```python
from build123d import *

# Parameters (mm, degrees)
ESBO_O1_W                   = 140
ESBO_O1_H                   = 95
RESSALTO_EXTRUS_O1_DEPTH    = 1.5
ESBO_O2_R                   = 1.5
ESBO_O2_W                   = 40
ESBO_O2_H                   = 3
CORTE_EXTRUS_O1_DEPTH       = 85.647799735
ESBO_O3_W                   = 3
ESBO_O3_H                   = 31
ESBO_O3_W_2                 = 30
ESBO_O3_H_2                 = 3
RESSALTO_EXTRUS_O2_DEPTH    = 3
CORTE_EXTRUS_O11_DEPTH      = 89.815820663
CORTE_EXTRUS_O11_DEPTH_BACK = 89.815820663
ESBO_O30_R                  = 4
CORTE_EXTRUS_O12_DEPTH      = 89.815820663
CORTE_EXTRUS_O12_DEPTH_BACK = 89.815820663
ESBO_O31_R                  = 1.5
CORTE_EXTRUS_O2_DEPTH       = 89.815820663
CUT_EXTRUDE2_DEPTH          = 89.777812543
CUT_EXTRUDE2_DEPTH_BACK     = 89.777812543
CUT_EXTRUDE6_DEPTH          = 89.815820663
CUT_EXTRUDE6_DEPTH_BACK     = 89.815820663
CUT_EXTRUDE8_DEPTH          = 89.777812543
CUT_EXTRUDE8_DEPTH_BACK     = 89.777812543
CUT_EXTRUDE9_DEPTH          = 89.815820663
CUT_EXTRUDE12_DEPTH         = 89.777812543
CUT_EXTRUDE12_DEPTH_BACK    = 89.777812543
SKETCH16_R                  = 1.5
FILLET1_R                   = 5


with BuildPart() as part:
    # Esboço1 → Ressalto-extrusão1 (new, symmetric)
    with BuildSketch(Plane.XY):
        Rectangle(ESBO_O1_W, ESBO_O1_H)
    extrude(amount=RESSALTO_EXTRUS_O1_DEPTH, both=True)

    # Esboço2 → Corte-extrusão1 (cut, through all)
    with BuildSketch(Plane.XY.offset(1.5)):
        with Locations((-31.5, -1)):
            Circle(ESBO_O2_R)
        with Locations(Location((31.5, -1, 0), (0, 0, 180))):
            Circle(ESBO_O2_R)
        with Locations((0, -46)):
            Rectangle(ESBO_O2_W, ESBO_O2_H)
        with Locations((0, -1)):
            Rectangle(ESBO_O2_W, ESBO_O2_H)
    extrude(amount=-CORTE_EXTRUS_O1_DEPTH, mode=Mode.SUBTRACT)

    # Esboço3 → Ressalto-extrusão2 (add, through all)
    with BuildSketch(Plane.XY.offset(1.5)):
        with Locations((71.5, 0)):
            Rectangle(ESBO_O3_W, ESBO_O3_H)
        with Locations((-71.5, 0)):
            Rectangle(ESBO_O3_W, ESBO_O3_H)
        with Locations((-35, 49)):
            Rectangle(ESBO_O3_W_2, ESBO_O3_H_2)
        with Locations((35, 49)):
            Rectangle(ESBO_O3_W_2, ESBO_O3_H_2)
    extrude(amount=-RESSALTO_EXTRUS_O2_DEPTH)

    # Esboço30 → Corte-extrusão11 (cut, two sides: drawn at the far end of the back side and taken through both)
    with BuildSketch(Plane(origin=(0, 0, -1.5), x_dir=(-1, 0, 0), z_dir=(0, 0, -1)).offset(-CORTE_EXTRUS_O11_DEPTH_BACK)):
        with Locations((55, -28.5)):
            Circle(ESBO_O30_R)
    extrude(amount=CORTE_EXTRUS_O11_DEPTH + CORTE_EXTRUS_O11_DEPTH_BACK, mode=Mode.SUBTRACT)

    # Esboço31 → Corte-extrusão12 (cut, two sides: drawn at the far end of the back side and taken through both)
    with BuildSketch(Plane(origin=(0, 0, -1.5), x_dir=(-1, 0, 0), z_dir=(0, 0, -1)).offset(-CORTE_EXTRUS_O12_DEPTH_BACK)):
        with Locations((64, -19.5)):
            Circle(ESBO_O31_R)
        with Locations((64, -37.5)):
            Circle(ESBO_O31_R)
        with Locations((31, -19.5)):
            Circle(ESBO_O31_R)
        with Locations((31, -37.5)):
            Circle(ESBO_O31_R)
    extrude(amount=CORTE_EXTRUS_O12_DEPTH + CORTE_EXTRUS_O12_DEPTH_BACK, mode=Mode.SUBTRACT)

    # Esboço4 → Corte-extrusão2 (cut, through all)
    with BuildSketch(Plane.XY.offset(1.5)):
        with BuildLine():
            Line((40, -26.5), (46, -26.5))
            ThreePointArc((46, -26.5), (48, -28.5), (46, -30.5))
            Line((46, -30.5), (40, -30.5))
            ThreePointArc((40, -30.5), (38, -28.5), (40, -26.5))
        make_face()
    extrude(amount=-CORTE_EXTRUS_O2_DEPTH, mode=Mode.SUBTRACT)

    # Sketch5 → Cut-Extrude2 (cut, two sides: drawn at the far end of the back side and taken through both)
    with BuildSketch(Plane.XY.offset(-CUT_EXTRUDE2_DEPTH_BACK)):
        with BuildLine():
            Line((-1.5, -44.5), (1.5, -44.5))
            Line((1.5, -44.5), (1.5, -40.5))
            Line((1.5, -40.5), (2.85, -40.5))
            Line((2.85, -40.5), (2.85, -38.23))
            Line((2.85, -38.23), (1.5, -38.23))
            Line((1.5, -38.23), (1.5, -33.5))
            ThreePointArc((1.5, -33.5), (1.207106781, -32.792893219), (0.5, -32.5))
            Line((0.5, -32.5), (-0.5, -32.5))
            ThreePointArc((-0.5, -32.5), (-1.207106781, -32.792893219), (-1.5, -33.5))
            Line((-1.5, -33.5), (-1.5, -38.23))
            Line((-1.5, -38.23), (-2.85, -38.23))
            Line((-2.85, -38.23), (-2.85, -40.5))
            Line((-2.85, -40.5), (-1.5, -40.5))
            Line((-1.5, -40.5), (-1.5, -44.5))
        make_face()
    extrude(amount=CUT_EXTRUDE2_DEPTH + CUT_EXTRUDE2_DEPTH_BACK, mode=Mode.SUBTRACT)

    # Sketch8 → Cut-Extrude6 (cut, two sides: drawn at the far end of the back side and taken through both)
    with BuildSketch(Plane.XY.offset(1.5).offset(-CUT_EXTRUDE6_DEPTH_BACK)):
        with BuildLine():
            Line((-56, 39.75), (-56, 26.75))
            ThreePointArc((-56, 26.75), (-56.439339828, 25.689339828), (-57.5, 25.25))
            Line((-57.5, 25.25), (-60.5, 25.25))
            ThreePointArc((-60.5, 25.25), (-61.560660172, 24.810660172), (-62, 23.75))
            Line((-62, 23.75), (-62, 23.5))
            ThreePointArc((-62, 23.5), (-63.5, 22), (-65, 23.5))
            Line((-65, 23.5), (-65, 23.75))
            ThreePointArc((-65, 23.75), (-65.24500996, 24.571583836), (-65.9, 25.124772708))
            ThreePointArc((-65.9, 25.124772708), (-66.336660027, 25.49356529), (-66.5, 26.041287847))
            Line((-66.5, 26.041287847), (-66.5, 40.458712153))
            ThreePointArc((-66.5, 40.458712153), (-66.336660027, 41.00643471), (-65.9, 41.375227292))
            ThreePointArc((-65.9, 41.375227292), (-65.24500996, 41.928416164), (-65, 42.75))
            Line((-65, 42.75), (-65, 43))
            ThreePointArc((-65, 43), (-63.5, 44.5), (-62, 43))
            Line((-62, 43), (-62, 42.75))
            ThreePointArc((-62, 42.75), (-61.560660172, 41.689339828), (-60.5, 41.25))
            Line((-60.5, 41.25), (-57.5, 41.25))
            ThreePointArc((-57.5, 41.25), (-56.439339828, 40.810660172), (-56, 39.75))
        make_face()
        with BuildLine():
            Line((56, 39.75), (56, 26.75))
            ThreePointArc((56, 26.75), (56.439339828, 25.689339828), (57.5, 25.25))
            Line((57.5, 25.25), (60.5, 25.25))
            ThreePointArc((60.5, 25.25), (61.560660172, 24.810660172), (62, 23.75))
            Line((62, 23.75), (62, 23.5))
            ThreePointArc((62, 23.5), (63.5, 22), (65, 23.5))
            Line((65, 23.5), (65, 23.75))
            ThreePointArc((65, 23.75), (65.24500996, 24.571583836), (65.9, 25.124772708))
            ThreePointArc((65.9, 25.124772708), (66.336660027, 25.49356529), (66.5, 26.041287847))
            Line((66.5, 26.041287847), (66.5, 40.458712153))
            ThreePointArc((66.5, 40.458712153), (66.336660027, 41.00643471), (65.9, 41.375227292))
            ThreePointArc((65.9, 41.375227292), (65.24500996, 41.928416164), (65, 42.75))
            Line((65, 42.75), (65, 43))
            ThreePointArc((65, 43), (63.5, 44.5), (62, 43))
            Line((62, 43), (62, 42.75))
            ThreePointArc((62, 42.75), (61.560660172, 41.689339828), (60.5, 41.25))
            Line((60.5, 41.25), (57.5, 41.25))
            ThreePointArc((57.5, 41.25), (56.439339828, 40.810660172), (56, 39.75))
        make_face()
    extrude(amount=CUT_EXTRUDE6_DEPTH + CUT_EXTRUDE6_DEPTH_BACK, mode=Mode.SUBTRACT)

    # Sketch11 → Cut-Extrude8 (cut, two sides: drawn at the far end of the back side and taken through both)
    with BuildSketch(Plane.XY.offset(-CUT_EXTRUDE8_DEPTH_BACK)):
        with BuildLine():
            Line((-36.5, 50.5), (-33.5, 50.5))
            Line((-33.5, 50.5), (-33.5, 46.5))
            Line((-33.5, 46.5), (-32.15, 46.5))
            Line((-32.15, 46.5), (-32.15, 44.23))
            Line((-32.15, 44.23), (-33.5, 44.23))
            Line((-33.5, 44.23), (-33.5, 39.5))
            ThreePointArc((-33.5, 39.5), (-33.792893219, 38.792893219), (-34.5, 38.5))
            Line((-34.5, 38.5), (-35.5, 38.5))
            ThreePointArc((-35.5, 38.5), (-36.207106781, 38.792893219), (-36.5, 39.5))
            Line((-36.5, 39.5), (-36.5, 44.23))
            Line((-36.5, 44.23), (-37.85, 44.23))
            Line((-37.85, 44.23), (-37.85, 46.5))
            Line((-37.85, 46.5), (-36.5, 46.5))
            Line((-36.5, 46.5), (-36.5, 50.5))
        make_face()
    extrude(amount=CUT_EXTRUDE8_DEPTH + CUT_EXTRUDE8_DEPTH_BACK, mode=Mode.SUBTRACT)

    # Sketch12 → Cut-Extrude9 (cut, through all)
    with BuildSketch(Plane.XY.offset(1.5)):
        with BuildLine():
            Line((-1.5, 20), (-1.5, 35))
            ThreePointArc((-1.5, 35), (0, 36.5), (1.5, 35))
            Line((1.5, 35), (1.5, 20))
            ThreePointArc((1.5, 20), (0, 18.5), (-1.5, 20))
        make_face()
    extrude(amount=-CUT_EXTRUDE9_DEPTH, mode=Mode.SUBTRACT)

    # Sketch16 → Cut-Extrude12 (cut, two sides: drawn at the far end of the back side and taken through both)
    with BuildSketch(Plane.XY.offset(-CUT_EXTRUDE12_DEPTH_BACK)):
        with Locations((-12.5, 15.35)):
            Circle(SKETCH16_R)
        with Locations((12.5, 15.35)):
            Circle(SKETCH16_R)
        with Locations((-12.5, -8.95)):
            Circle(SKETCH16_R)
        with Locations((12.5, -8.95)):
            Circle(SKETCH16_R)
        with BuildLine():
            Line((10.5, 13.35), (14.5, 13.35))
            ThreePointArc((14.5, 13.35), (15.207106781, 13.057106781), (15.5, 12.35))
            Line((15.5, 12.35), (15.5, 4.15))
            ThreePointArc((15.5, 4.15), (15.207106781, 3.442893219), (14.5, 3.15))
            Line((14.5, 3.15), (10.5, 3.15))
            ThreePointArc((10.5, 3.15), (9.792893219, 3.442893219), (9.5, 4.15))
            Line((9.5, 4.15), (9.5, 12.35))
            ThreePointArc((9.5, 12.35), (9.792893219, 13.057106781), (10.5, 13.35))
        make_face()
    extrude(amount=CUT_EXTRUDE12_DEPTH + CUT_EXTRUDE12_DEPTH_BACK, mode=Mode.SUBTRACT)

    # Fillet1
    fillet1_edges = [part.edges().sort_by_distance(p)[0] for p in [
        (-70, 47.5, 0),
        (70, 47.5, 0),
    ]]
    fillet(fillet1_edges, radius=FILLET1_R)


solid = part.part
```
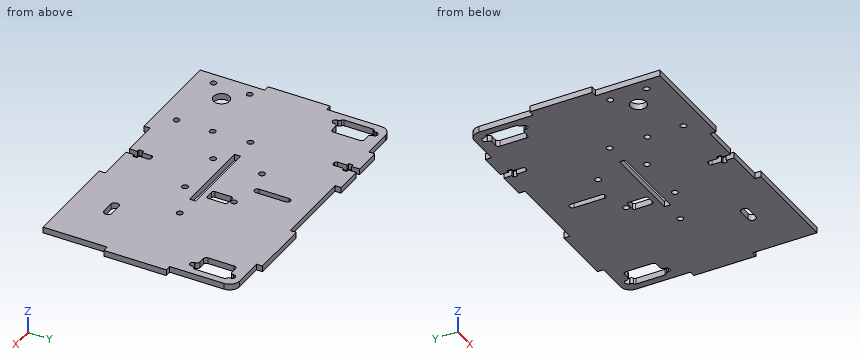
Geometry: final body of the model. Coordinates: model frame, mm. Round coordinates to 2 decimals unless told otherwise and drop trailing zeros. Order: outer loops, then holes, each group sorted by start corner. A loop starts at its lowest first (then second) coordinate and runs counter-clockwise, first axis right, second up. Notation, with made-up numbers: M -25,40.5 L -18,40.5 A32 ccw -18,71.5 Z; hole C 71,64.25 d11. An arc over 180 degrees is marked long. Use one line per item in the form item = value. Start each with the question number.
Q1. Cut plane D-D (z = -0.7). Count the separate pieces of the cut face and the enclosed holes in it, and give its area (3 significant figures).
Q2. Pin query (flat end, axial travel): pin 1 Ø0.9 at (y, z) = (42.5, 0) entering from +X; pin 2 Ø1.1 at (x, z) = (0, 0) entering from -Y; pin 3 Ø1.5 at (y, z) = (49, 0) entering from -X. Return the tip coordinate at first contact, or that it passes through.
Q3. Cut plane A-A (y = -28.5). Return loops of the section in (x, z), and give its area (3 significant figures).
Q4. Cut plane C-C (x = -12.5). Return loops of the section in (y, z).
Q5. Cut plane B-B (x = 42). Return loops of the section in (y, z).
Q6. Material intervals for line 1 (X direction, y = -8.95, z = 0.25); line 2 (X direction, y = 34, z = -1.1); line 3 (Y direction, x = -6.5, z = 0.3), sorted ascending. Write a range as [from, to].
Geometry results:
q1.separate_pieces = 1
q1.enclosed_holes = 17
q1.area = 12,700 mm^2
q2.pin_1 = 70
q2.pin_2 = -32.5
q2.pin_3 = -50
q3.outline = M -70,-1.5 L -59,-1.5 L -59,1.5 L -70,1.5 Z; M -51,-1.5 L 38,-1.5 L 38,1.5 L -51,1.5 Z; M 48,-1.5 L 70,-1.5 L 70,1.5 L 48,1.5 Z
q3.area = 366 mm^2
q4.outline = M -44.5,-1.5 L -10.45,-1.5 L -10.45,1.5 L -44.5,1.5 Z; M -7.45,-1.5 L -2.5,-1.5 L -2.5,1.5 L -7.45,1.5 Z; M 0.5,-1.5 L 13.85,-1.5 L 13.85,1.5 L 0.5,1.5 Z; M 16.85,-1.5 L 47.5,-1.5 L 47.5,1.5 L 16.85,1.5 Z
q5.outline = M -47.5,-1.5 L -30.5,-1.5 L -30.5,1.5 L -47.5,1.5 Z; M -26.5,-1.5 L 50.5,-1.5 L 50.5,1.5 L -26.5,1.5 Z
q6.line_1 = [-73, -14], [-11, 11], [14, 73]
q6.line_2 = [-70, -66.5], [-56, -1.5], [1.5, 56], [66.5, 70]
q6.line_3 = [-44.5, -2.5], [0.5, 47.5]
